Can you work these out from the model? Positions are in its coordinate system, mm. Face numbers are marked on the shaded views. A direction names the side the tool comes from. Coordinates: 2 decimals unless noted, no trailing zeros. Write each loop counter-clockwise with the first axis right and the second up, starting at its lowest first coordinate (ties: lowest second). Pieces come first, ordered by that corner, then holes. Notation, with made-up numbers: M 59.25,46.5 L 66.25,46.5 A25 ccw 66.25,75.5 Z; hole C 40.25,-39 d3. An arc over 180 degrees is marked long. Answer as a JSON object with one key per item and string values. Group by question number.
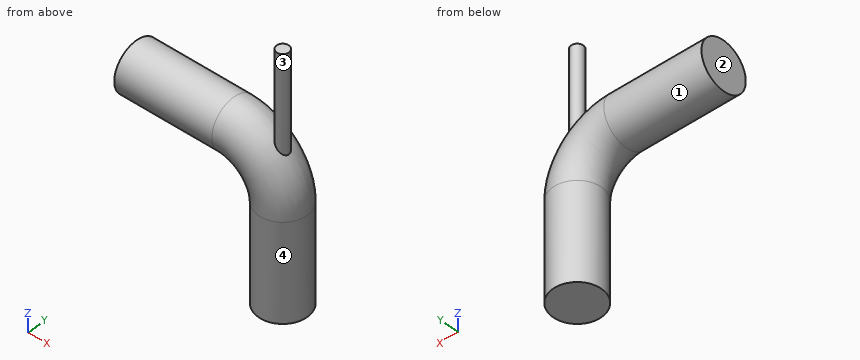
from build123d import *

# Parameters (mm, degrees)
F1_R = 160
F4_R = 40


with BuildPart() as f2:
    # F2: sweep along a path in F0
    with BuildLine(Plane.XZ) as f2_path:
        Line((-640, 0), (0, 0))
        ThreePointArc((0, 0), (226.2741699797, -93.7258300203), (320, -320))
        Line((320, -320), (320, -960))
    # F1 (on Right) → F2 (sweep)
    with BuildSketch(Plane.YZ):
        Circle(F1_R)
    sweep(path=f2_path.line)

    # F5: sweep along a path in F3
    with BuildLine(Plane.XZ) as f5_path:
        Line((320, 640), (320, -183.2472234964))
    # F4 (on Top) → F5 (sweep)
    with BuildSketch(Plane.XY):
        with Locations((320, 0)):
            Circle(F4_R)
    sweep(path=f5_path.line)


solid = f2.part
Q1. If we section it at C-C on y = 0: List the corners of the cut face in (x, z) for me, and give its area (3 significant figures).
Q2. If we section it at B-B on z = -449: List the corners of the cut face in (x, y) for me, and give its area (3 significant figures).
Q3. Will these pins go through, and if not, where does the flat tip stop? pin 1 (1.5 mm diameter, centred on y = -55.5, z = -364.5, fed in from +X); pin 2 (12 mm diameter, centred on x = 53, y = 103.5, fed in from -Z); pin 3 (2 mm diameter, centred on x = -495.5, y = -31, fed in from +Z).
Q4. On a 3-axis mill with a long thin cutter (end or side, diameter ignored), from which of +Z, -Z, +X, -X, +Y, -Y can I reach the whole of each face in a straight line? I mean the marked faces 1, 2, 3 and 4. Say none if no direction works.
Q5. If we section it at A-A on x = -91.5: List the corners of the cut face in (y, z) for me.
Q6. Please list where these lines run through material, in increasing order: L1, parallel to X at y = -4, z = 263; L2, parallel to X at y = 13.5, z = 48; L3, parallel to Z at x = -582, y = -125.5.
Reply:
{
 "1": {"outline": "M -640,-160 L 0,-160 A160 cw 160,-320 L 160,-960 L 480,-960 L 480,-320 A480 ccw 360,-2.51 L 360,640 L 280,640 L 280,69.87 A480 ccw 0,160 L -640,160 Z", "area": "619,000 mm^2"},
 "2": {"outline": "C 320,0 d320", "area": "80,400 mm^2"},
 "3": {"pin 1": "x = 470.34", "pin 2": "z = -134.58", "pin 3": "z = 157.16"},
 "4": {"face 1": "-X", "face 2": "+Z, -Z, -X, +Y, -Y", "face 3": "+Z", "face 4": "-Z"},
 "5": {"outline": "C 0,0 d320"},
 "6": {"L1": "280.2 to 359.8", "L2": "-640 to 357.65", "L3": "-99.25 to 99.25"}
}
